Model file for the job. Use its own axes, mm. A direction names the side the tool comes from. Give positions to 0.01 mm unless a question says otherwise; leave off trailing zeros. Loops run counter-clockwise (first coordinate to the right, second up) from the corner with the lowest first, then second, coordinate; pieces in that order, holes last. Notation, with made-up numbers: M 82.5,57.5 L 90.5,57.5 A12 cw 90.5,72.5 Z; hole C 50.5,-36.75 d7. An arc over 180 degrees is marked long. Answer in a Markdown table with one row per item.
Autodesk Inventor part; units mm, degrees
ref_plane "РабПлоскость4" through (0, 0, 0) normal (0, 0, -1) x (-1, 0, 0)
ref_plane "РабПлоскость2" through (0, 0, 7) normal (0, 0, 1) x (1, 0, 0)
ref_plane "YZ Plane" through (0, 0, 0) normal (1, 0, 0) x (0, 1, 0)
sketch "Эскиз1" plane through (0, 0, 0) normal (0, 0, 1) x (1, 0, 0)
  circle A0 centre (0, 0) radius 6.75
  circle A1 centre (0, 0) radius 3.05
  dimension "d0" = 13.5
  dimension "d1" = 6.1
ref_plane "РабПлоскость1" through (0, 0, 35) normal (0, 0, 1) x (1, 0, 0)
sketch "Эскиз2" plane through (0, 0, 35) normal (0, 0, 1) x (1, 0, 0)
  circle A0 centre (0, 0) radius 15.75
  dimension "d5" = 31.5
extrude "Выдавливание2" add sketch "Эскиз2" against normal blind 3
sketch "Эскиз3" plane through (0, 0, 35) normal (0, 0, 1) x (1, 0, 0)
  line L0 (0, 0) -> (0, 11.319)
  line L1 (0, 0) -> (11.319, 0) construction
  circle A0 centre (0, 11.319) radius 2.2
  circle A1 centre (0, 0) radius 1.4142
  circle A2 centre (-8.0037, 8.0037) radius 2.2
  circle A3 centre (-11.319, 0) radius 2.2
  circle A4 centre (-8.0037, -8.0037) radius 2.2
  circle A5 centre (0, -11.319) radius 2.2
  circle A6 centre (8.0037, -8.0037) radius 2.2
  circle A7 centre (11.319, 0) radius 2.2
  circle A8 centre (8.0037, 8.0037) radius 2.2
  dimension "d8" = 11.319
  dimension "d9" = 90
  dimension "d10" = 4.4
  dimension "d13" = 360
extrude "Выдавливание3" cut sketch "Эскиз3" against normal blind 3 contours A0 | A2 | A3 | A4 | A5 | A6 | A7 | A8
ref_plane "РабПлоскость4" through (0, 0, 0) normal (0, 0, -1) x (-1, 0, 0)
sketch "Эскиз4" plane through (0, 0, 0) normal (0, 0, -1) x (-1, 0, 0)
  circle A0 centre (0, 0) radius 13.15
  circle A1 centre (0, 0) radius 9.5
  dimension "d17" = 26.3
  dimension "d18" = 19
extrude "Выдавливание4" add sketch "Эскиз4" against normal blind 10
ref_plane "РабПлоскость2" through (0, 0, 7) normal (0, 0, 1) x (1, 0, 0)
ref_plane "РабПлоскость3" through (0, 0, 47.5) normal (0, 0, 1) x (1, 0, 0)
sketch "Эскиз6" plane through (0, 0, 47.5) normal (0, 0, 1) x (1, 0, 0)
  circle A0 centre (0, 0) radius 6.75
  circle A1 centre (0, 0) radius 3.05
  dimension "d28" = 13.5
  dimension "d29" = 6.1
ref_plane "РабПлоскость5" through (0, 0, 6) normal (0, 0, 1) x (1, 0, 0)
sketch "Эскиз7" plane through (0, 0, 6) normal (0, 0, 1) x (1, 0, 0)
  circle A0 centre (0, 0) radius 7.5
  circle A1 centre (0, 0) radius 9.5
  dimension "d31" = 15
  dimension "d32" = 19
extrude "Выдавливание7" add sketch "Эскиз7" along normal blind 4 contours A0 | A1
extrude "Выдавливание8" cut sketch "Эскиз7" along normal blind 1 contours A0
extrude "Выдавливание9" add sketch "Эскиз6" against normal blind 38.5
properties part number "Затычка для Косозубки"
(1) Flat gauge pins, fed straight in: P1, Ø5.5, axis at x = -4.5, y = 2.5, coming from the -Z side; P2, Ø5, axis at x = 10.5, z = 13.5, coming from the -Y side; P3, Ø1.5, axis at x = 8, y = -4, coming from the +Z side; P4, Ø4, axis at x = -2.5, z = 35, coming from the +Y side. Where does each tip first touch, or does it go through?
Established:
| item | result |
|---|---|
| P1 | stops at z = 6 |
| P2 | passes through |
| P3 | stops at z = 35 |
| P4 | stops at y = 15.74 |
(2) Mould opens along X. For faces 5 (the cylindrical face through (-4.38, -8.43, 2.96)), 6 (the flat face through (2.9, -1.4, 47.5)), 7 (the cylindrical face through (13.137, 0.578, 4.93)) say: pulls with the +X half, pulls with the -X half, needs draft (parallel to the pull), parting line crosses it, or undercut.
Established:
| item | result |
|---|---|
| face 5 | undercut |
| face 6 | needs draft |
| face 7 | parting line crosses it |
(3) Saw through at D-D, the plane y = -4.5. Give the cut face in (x, z).
Established:
| item | result |
|---|---|
| outline | M -15.09,32 L -5.03,32 L -5.03,10 L -12.36,10 L -12.36,0 L -8.37,0 L -8.37,6 L -6,6 L -6,7 L 6,7 L 6,6 L 8.37,6 L 8.37,0 L 12.36,0 L 12.36,10 L 5.03,10 L 5.03,32 L 15.09,32 L 15.09,35 L 5.03,35 L 5.03,47.5 L -5.03,47.5 L -5.03,35 L -15.09,35 Z |
(4) Saw through at C-C, the plane z = 37.5. Give the cut face in (x, y).
Established:
| item | result |
|---|---|
| outline | C 0,0 d13.5; hole C 0,0 d6.1 |
(5) Saw through at A-A, the plane y = 0. Count the separate pieces of the cut face and the enclosed holes in it, and give its area (3 significant figures).
Established:
| item | result |
|---|---|
| separate pieces | 3 |
| enclosed holes | 1 |
| area | 457 mm2 |
(6) Which spindle directions (+Z, -Z, +X, -X, +Y, -Y) get a long thin tool onto all of the face, cutting with end or side? Do faces 1 (the flat face through (-4, -9, 0)), 2 (the flat face through (1, 8, 6)), 3 (the flat face through (7, 0, 32)), 4 (the cylindrical face through (-3.047, 0.134, 41.338)). Say none if no direction does.
Established:
| item | result |
|---|---|
| face 1 | -Z, +X, -X, +Y, -Y |
| face 2 | -Z |
| face 3 | none |
| face 4 | +Z |
(7) Wall check: L1, parallel to Y at x = 0, z = 32.8; L2, parallel to Y at x = 0, z = 24.25; L3, parallel to Z at x = 3.5, y = -12.5. Give the ranges that are in metal, low to high.
Established:
| item | result |
|---|---|
| L1 | y = -15.75 to -13.52, -9.12 to 9.12, 13.52 to 15.75 |
| L2 | y = -6.75 to -3.05, 3.05 to 6.75 |
| L3 | z = 0 to 10, 32 to 35 |
